Autodesk Inventor part; units mm, degrees
ref_plane "YZ Plane" through (0, 0, 0) normal (1, 0, 0) x (0, 1, 0)
ref_plane "XZ Plane" through (0, 0, 0) normal (0, 1, 0) x (-1, 0, 0)
ref_plane "XY Plane" through (0, 0, 0) normal (0, 0, 1) x (1, 0, 0)
sketch "Sketch1" plane through (0, 0, 0) normal (0, 0, 1) x (1, 0, 0)
  line L0 (-19, 0) -> (19, 0) construction
  line L1 (-19, -2.25) -> (19, -2.25)
  line L2 (19, 2.25) -> (-19, 2.25)
  arc A0 (-19, 2.25) -> (-19, -2.25) centre (-19, 0) ccw
  arc A1 (19, -2.25) -> (19, 2.25) centre (19, 0) ccw
  circle A2 centre (-19, 0) radius 1.35
  point P0 (0, 0)
  dimension "d0" = 4.5
  dimension "d1" = 38
  dimension "d8" = 2.7
extrude "Extrusion1" add sketch "Sketch1" along normal mid plane 10
sketch "Sketch2" plane through (-19, 2.25, -5) normal (0, 1, 0) x (1, 0, 0)
  line L0 (-8.25, -7.5) -> (3.75, -7.5)
  line L1 (3.75, -7.5) -> (3.75, -2.5)
  line L2 (3.75, -2.5) -> (-8.25, -2.5)
  line L3 (-8.25, -2.5) -> (-8.25, -7.5)
  line L4 (-2.25, 0) -> (-2.25, -10)
  line L5 (-8.25, -7.5) -> (3.75, -2.5) construction
  line L6 (3.75, -7.5) -> (-8.25, -2.5) construction
  point P0 (19, -5)
  point P1 (-2.25, -5)
  dimension "d4" = 5
  dimension "d5" = 6
extrude "Extrusion2" cut sketch "Sketch2" against normal through all
sketch "Sketch3" plane through (-19, 2.25, -5) normal (0, 1, 0) x (1, 0, 0)
  line L0 (1.35, -10) -> (-1.35, -10) construction
  line L1 (-1.35, 0) -> (1.35, 0) construction
  line L2 (0, -7.5) -> (0, -10) construction
  line L3 (0, -10) -> (0, 0) construction
  line L4 (0, -5) -> (34.5, -5) construction
  line L5 (35.5, -5) -> (33.5, -5) construction
  line L6 (35.5, -3) -> (33.5, -3)
  line L7 (33.5, -7) -> (35.5, -7)
  arc A0 (35.5, -7) -> (35.5, -3) centre (35.5, -5) ccw
  arc A1 (33.5, -3) -> (33.5, -7) centre (33.5, -5) ccw
  point P0 (19, -5)
  dimension "d9" = 34.5
  dimension "d11" = 2
  dimension "d12" = 2
extrude "Extrusion3" cut sketch "Sketch3" against normal through all
sketch "Sketch4" plane through (0, 0, 0) normal (0, 0, 1) x (1, 0, 0)
  line L0 (-19, -2.25) -> (19, -2.25)
  line L1 (-2.75, -2.25) -> (-2.75, -7.25)
  line L2 (-3.6897, -6.592) -> (-5.2701, -2.25)
  arc A0 (-3.6897, -6.592) -> (-2.75, -7.25) centre (-2.75, -6.25) ccw
  circle A1 centre (-19, 0) radius 1.35
  point P0 (0, 0)
  dimension "d15" = 1
  dimension "d16" = 70
  dimension "d18" = 16.25
  dimension "d21" = 5
revolve "Revolution1" add sketch "Sketch4" angle 360 about axis through (-2.75, -2.25, 0) along (0, -1, 0) contours L0 L1 A0 L2
sketch "Sketch5" plane through (-19, 2.25, 5) normal (0, 1, 0) x (1, 0, 0)
  line L0 (42.5072, 5) -> (-11.8612, 5)
  line L1 (-11.8612, 5) -> (-11.8612, 14.1834)
  line L2 (-11.8612, 14.1834) -> (42.5072, 14.1834)
  line L3 (42.5072, 14.1834) -> (42.5072, 5)
  point P0 (19, 5)
properties part number "RegulatorHinge"
Geometry check sheet. Reference: the model listing, model coordinates, mm. A direction names the side the tool comes from. Round coordinates to 2 decimals unless told otherwise and drop trailing zeros. Loops run counter-clockwise (first coordinate to the right, second up) from the corner with the lowest first, then second, coordinate; pieces in that order, holes last.
Item 1: Access from +Z, -Z, +X, -X, +Y, -Y to the whole of each face (thin tool, end or side, straight path). Record for faces 1 (the flat face through (-17, 0, 2.5)), 2 (the cylindrical face through (18.5, 0, 0)), 3 (the cylindrical face through (21.25, 0.05, -0.07)).
Item 2: Mould release check, pull along X, two halves, no side actions. Record for faces 4 (the conical face through (-2.41, -4.87, -1.53)), 5 (the cylindrical face through (-17.712, -0.406, 3.732)), 6 (the flat face through (0, 2.25, 0)): pulls with the +X half, pulls with the -X half, needs draft (parallel to the pull), parting line crosses it, or undercut.
Item 3: Cross-section at D-D on y = -4. Record the boundary of the cut face in (x, z).
Item 4: Gauge pin test, flat ends, axial feed: pin 1 (1 mm diameter, centred on x = 6, z = -1.5, fed in from -Y); pin 2 (2 mm diameter, centred on x = -19.5, y = 0.5, fed in from +Z); pin 3 (4 mm diameter, centred on y = -5, z = -1, fed in from -X); pin 4 (1.3 mm diameter, centred on y = 0, z = -1, fed in from -X). Record the tip position at first contact, or that the pin passes through.
Item 5: Cross-section at A-A on y = -0.5. Record the boundary of the cut face in (x, z), then the cut area to 3 significant figures.
Item 6: Cross-section at B-B on x = 18. Record the boundary of the cut face in (y, z), then the cut area to 3 significant figures.
Item 7: Cross-section at C-C on x = 9. Record the boundary of the cut face in (y, z).
Item 8: Thickness scan on line 1 (Y direction, x = -19, z = -3.1); line 2 (X direction, y = 0, z = -3.45); line 3 (Y direction, x = -10.5, z = -1.5). Record the ranges inside material, lowest first.
Answer sheet:
1. face 1: -X, +Y, -Y
1. face 2: +Y, -Y
1. face 3: +Z, -Z, +X
2. face 4: parting line crosses it
2. face 5: undercut
2. face 6: needs draft
3. outline: circle Ø3.77 at (-2.75, 0)
4. pin 1: stops at y = -2.25
4. pin 2: stops at z = 5
4. pin 3: stops at x = -4.93
4. pin 4: stops at x = -15.25
5. outline: (-21.19, -5) - (-20.25, -5) - (-20.25, -2.5) - (-21.19, -2.5) - close; (-21.19, 2.5) - (-20.25, 2.5) - (-20.25, 5) - (-21.19, 5) - close; (-17.75, -5) - (21.19, -5) - (21.19, 5) - (-17.75, 5) - (-17.75, 2.5) - (-15.25, 2.5) - (-15.25, -2.5) - (-17.75, -2.5) - close; hole (14.5, -2) - (16.5, -2) arc R2 ccw to (16.5, 2) - (14.5, 2) arc R2 ccw to start
5. area: 361 mm2
6. outline: (-2.25, -5) - (2.25, -5) - (2.25, -1.32) - (-2.25, -1.32) - close; (-2.25, 1.32) - (2.25, 1.32) - (2.25, 5) - (-2.25, 5) - close
6. area: 33.1 mm2
7. outline: (-2.25, -5) - (2.25, -5) - (2.25, 5) - (-2.25, 5) - close
8. line 1: y = -2.25 to -1.35, 1.35 to 2.25
8. line 2: x = -21.25 to -20.35, -17.65 to 21.25
8. line 3: y = -2.25 to 2.25
